Check sheet for the modelled part. Datum: model origin and axes. Units: mm. Coordinates: 2 decimals unless noted, no trailing zeros. Loops run counter-clockwise (first coordinate to the right, second up) from the corner with the lowest first, then second, coordinate; pieces in that order, holes last. Notation, with made-up numbers: M 51,56.5 L 107,56.5 A7 ccw 107,64.5 Z; hole C -32,-12.75 d5. An arc over 180 degrees is marked long. Use CSV: the item, a comma, the result in double quotes. Start each with the question number.
(1) Section check C-C on x = 0. Record the cut outline in (y, z).
(2) Section check A-A on x = -3.81. Record the cut outline in (y, z), and give its area (3 significant figures).
(3) Section check B-B on z = 2.25. Record the cut outline in (x, y).
(4) Draft check along X on faces 1 (the flat face through (-1, 0, 0)), 2 (the cylindrical face through (-2.16, -0.49, 3.77)), 3 (the flat face through (-5.48, -0.5, 0.1)). Enter one of: pulls with the +X half, pulls with the -X half, needs draft (parallel to the pull), parting line crosses it, or undercut.
(5) Section check D-D on y = -0.7. Give the number of separate pieces and of enclosed holes in the cut face, and give its area (3 significant figures).
(6) Scan lines: line 1 (Z direction, x = -3.81, y = -0.6); line 2 (Z direction, x = 0, y = -0.6); line 3 (X direction, y = -0.1, z = -3.75). Record each from-to range of solid material in increasing order.
from build123d import *

# Parameters (mm, degrees)
F0_R     = 0.4
F0_W     = 4.21
F0_H     = 2.54
F1_DEPTH = 1


# Not quite as in the source:
# - ends of sketch curves that miss each other by under 0.0002 mm in the source are joined


with BuildPart() as f1:
    # F0 (on Front) → F1 (new body)
    with BuildSketch(Plane.XZ):
        with BuildLine():
            Line((4.153313, 2.713934), (2.1644269248, 3.7083768497))
            Line((2.1644269248, 3.7083768497), (-0.77, 3.708377))
            ThreePointArc((-0.77, 3.708377), (-1.1235533906, 3.5619303906), (-1.27, 3.208377))
            Line((-1.27, 3.208377), (-1.27, 2.438377))
            Line((-1.27, 2.438377), (-1.27, -0.101623))
            Line((-1.27, -0.101623), (5.48, -0.101623))
            Line((5.48, -0.101623), (5.48, 0.567309))
            ThreePointArc((5.48, 0.567309), (5.1215620576, 1.8290634789), (4.153313, 2.713934))
        make_face()
        with Locations((0, 1.168377)):
            Circle(F0_R, mode=Mode.SUBTRACT)
        with Locations((1.27, 1.168377)):
            Circle(F0_R, mode=Mode.SUBTRACT)
        with Locations((2.54, 1.168377)):
            Circle(F0_R, mode=Mode.SUBTRACT)
        with Locations((0, 2.438377)):
            Circle(F0_R, mode=Mode.SUBTRACT)
        with Locations((1.27, 2.438377)):
            Circle(F0_R, mode=Mode.SUBTRACT)
        with Locations((3.81, 1.168377)):
            Circle(F0_R, mode=Mode.SUBTRACT)
        with Locations((3.130691, 2.25)):
            Circle(F0_R, mode=Mode.SUBTRACT)
        with BuildLine():
            Line((2.1644269248, 3.7083768497), (-1.13809, 5.359635))
            ThreePointArc((-1.13809, 5.359635), (-1.1815821983, 5.3753997465), (-1.227533, 5.38075))
            Line((-1.227533, 5.38075), (-5.28, 5.38075))
            ThreePointArc((-5.28, 5.38075), (-5.4214213562, 5.3221713562), (-5.48, 5.18075))
            Line((-5.48, 5.18075), (-5.48, 2.438377))
            Line((-5.48, 2.438377), (-1.27, 2.438377))
            Line((-1.27, 2.438377), (-1.27, 3.208377))
            ThreePointArc((-1.27, 3.208377), (-1.1235533906, 3.5619303906), (-0.77, 3.708377))
            Line((-0.77, 3.708377), (2.1644269248, 3.7083768497))
        make_face()
        with Locations((-3.81, 3.708377)):
            Circle(F0_R, mode=Mode.SUBTRACT)
        with Locations((-2.54, 3.65085)):
            Circle(F0_R, mode=Mode.SUBTRACT)
        with Locations((-3.375, 1.168377)):
            Rectangle(F0_W, F0_H)
        with Locations((-3.81, 1.168377)):
            Circle(F0_R, mode=Mode.SUBTRACT)
        with Locations((-2.54, 1.168377)):
            Circle(F0_R, mode=Mode.SUBTRACT)
        with Locations((-3.375, -1.371623)):
            Rectangle(F0_W, F0_H)
        with Locations((-3.81, -1.371623)):
            Circle(F0_R, mode=Mode.SUBTRACT)
        with Locations((-2.486643, -1.406452)):
            Circle(F0_R, mode=Mode.SUBTRACT)
        with BuildLine():
            Line((-1.27, -3.411623), (-1.27, -2.641623))
            Line((-1.27, -2.641623), (-5.48, -2.641623))
            Line((-5.48, -2.641623), (-5.48, -5.18075))
            ThreePointArc((-5.48, -5.18075), (-5.4214213562, -5.3221713562), (-5.28, -5.38075))
            Line((-5.28, -5.38075), (-0.773828, -5.38075))
            Line((-0.773828, -5.38075), (2.1644269193, -3.9116228385))
            Line((2.1644269193, -3.9116228385), (-0.77, -3.911623))
            ThreePointArc((-0.77, -3.911623), (-1.1235533906, -3.7651763906), (-1.27, -3.411623))
        make_face()
        with Locations((-3.81, -3.911623)):
            Circle(F0_R, mode=Mode.SUBTRACT)
        with Locations((-2.54, -3.911623)):
            Circle(F0_R, mode=Mode.SUBTRACT)
        with BuildLine():
            Line((5.48, -0.770555), (5.48, -0.101623))
            Line((5.48, -0.101623), (-1.27, -0.101623))
            Line((-1.27, -0.101623), (-1.27, -2.641623))
            Line((-1.27, -2.641623), (-1.27, -3.411623))
            ThreePointArc((-1.27, -3.411623), (-1.1235533906, -3.7651763906), (-0.77, -3.911623))
            Line((-0.77, -3.911623), (2.164427, -3.911623))
            Line((2.164427, -3.911623), (4.153313, -2.91718))
            ThreePointArc((4.153313, -2.91718), (5.1215620576, -2.0323094789), (5.48, -0.770555))
        make_face()
        with Locations((0, -2.641623)):
            Circle(F0_R, mode=Mode.SUBTRACT)
        with Locations((1.27, -2.641623)):
            Circle(F0_R, mode=Mode.SUBTRACT)
        with Locations((0, -1.371623)):
            Circle(F0_R, mode=Mode.SUBTRACT)
        with Locations((1.27, -1.371623)):
            Circle(F0_R, mode=Mode.SUBTRACT)
        with Locations((2.54, -1.371623)):
            Circle(F0_R, mode=Mode.SUBTRACT)
        with Locations((3.220234, -2.503932)):
            Circle(F0_R, mode=Mode.SUBTRACT)
        with Locations((3.81, -1.371623)):
            Circle(F0_R, mode=Mode.SUBTRACT)
    extrude(amount=F1_DEPTH)


solid = f1.part
Outcome:
1,outline,"M -1,-4.99 L 0,-4.99 L 0,-3.04 L -1,-3.04 Z; M -1,-2.24 L 0,-2.24 L 0,-1.77 L -1,-1.77 Z; M -1,-0.97 L 0,-0.97 L 0,0.77 L -1,0.77 Z; M -1,1.57 L 0,1.57 L 0,2.04 L -1,2.04 Z; M -1,2.84 L 0,2.84 L 0,4.79 L -1,4.79 Z"
2,outline,"M -1,-5.38 L 0,-5.38 L 0,-4.31 L -1,-4.31 Z; M -1,-3.51 L 0,-3.51 L 0,-1.77 L -1,-1.77 Z; M -1,-0.97 L 0,-0.97 L 0,0.77 L -1,0.77 Z; M -1,1.57 L 0,1.57 L 0,3.31 L -1,3.31 Z; M -1,4.11 L 0,4.11 L 0,5.38 L -1,5.38 Z"
2,area,"7.56 mm²"
3,outline,"M -5.48,-1 L -0.35,-1 L -0.35,0 L -5.48,0 Z; M 0.35,-1 L 0.92,-1 L 0.92,0 L 0.35,0 Z; M 1.62,-1 L 2.73,-1 L 2.73,0 L 1.62,0 Z; M 3.53,-1 L 4.79,-1 L 4.79,0 L 3.53,0 Z"
4,face 1,"needs draft"
4,face 2,"undercut"
4,face 3,"pulls with the -X half"
5,separate pieces,"1"
5,enclosed holes,"22"
5,area,"85.3 mm²"
6,line 1,"z = -5.38 to -4.31, -3.51 to -1.77, -0.97 to 0.77, 1.57 to 3.31, 4.11 to 5.38"
6,line 2,"z = -4.99 to -3.04, -2.24 to -1.77, -0.97 to 0.77, 1.57 to 2.04, 2.84 to 4.79"
6,line 3,"x = -5.48 to -4.18, -3.44 to -2.91, -2.17 to 2.49"
